Model file for the job. Use its own axes, mm. Round coordinates to 2 decimals unless told otherwise and drop trailing zeros. Loops run counter-clockwise (first coordinate to the right, second up) from the corner with the lowest first, then second, coordinate; pieces in that order, holes last. Notation, with made-up numbers: (22, 25.25) - (62, 25.25) arc R21 cw to (62, 57.25) - close; hole circle Ø10 at (-10.5, 49.25). An arc over 180 degrees is marked (long way). Use one line per item in the form item = value.
from build123d import *

# Parameters (mm, degrees)
SKETCH1_W           = 132
SKETCH1_H           = 87
BOSS_EXTRUDE1_DEPTH = 2
SKETCH2_W           = 80
SKETCH2_H           = 55
BOSS_EXTRUDE2_DEPTH = 2
SKETCH3_W           = 76
SKETCH3_H           = 51
CUT_EXTRUDE1_DEPTH  = 2
SKETCH4_W           = 70
SKETCH4_H           = 45
CUT_EXTRUDE2_DEPTH  = 2


with BuildPart() as part:
    # Sketch1 → Boss-Extrude1 (new body)
    with BuildSketch(Plane(origin=(0, 0, 0), x_dir=(1, 0, 0), z_dir=(0, 1, 0))):
        Rectangle(SKETCH1_W, SKETCH1_H)
    extrude(amount=BOSS_EXTRUDE1_DEPTH)

    # Sketch2 → Boss-Extrude2 (add)
    with BuildSketch(Plane(origin=(0, 2, 0), x_dir=(1, 0, 0), z_dir=(0, 1, 0))):
        Rectangle(SKETCH2_W, SKETCH2_H)
    extrude(amount=BOSS_EXTRUDE2_DEPTH)

    # Sketch3 → Cut-Extrude1 (cut)
    with BuildSketch(Plane(origin=(0, 4, 0), x_dir=(1, 0, 0), z_dir=(0, 1, 0))):
        Rectangle(SKETCH3_W, SKETCH3_H)
    extrude(amount=-CUT_EXTRUDE1_DEPTH, mode=Mode.SUBTRACT)

    # Sketch4 → Cut-Extrude2 (cut)
    with BuildSketch(Plane(origin=(0, 2, 0), x_dir=(1, 0, 0), z_dir=(0, 1, 0))):
        Rectangle(SKETCH4_W, SKETCH4_H)
    extrude(amount=-CUT_EXTRUDE2_DEPTH, mode=Mode.SUBTRACT)


solid = part.part
1. Wall check: probe 1 along Z at (x, y) = (27, 1.55); probe 2 along Z at (x, y) = (22.5, 3.1); probe 3 along X at (y, z) = (2.65, -4.5). Give the ranges that are in metal, low to high.
Geometry check:
probe_1 = -43.5 to -22.5, 22.5 to 43.5
probe_2 = -27.5 to -25.5, 25.5 to 27.5
probe_3 = -40 to -38, 38 to 40
2. Cut at D-D, the plane z = 24. Give the cut face in (x, y), plus the area to 3 significant figures.
Geometry check:
outline = (-66, 0) - (66, 0) - (66, 2) - (40, 2) - (40, 4) - (38, 4) - (38, 2) - (-38, 2) - (-38, 4) - (-40, 4) - (-40, 2) - (-66, 2) - close
area = 272 mm^2
3. Cut at A-A, the plane z = 1. Give the cut face in (x, y), plus the area to 3 significant figures.
Geometry check:
outline = (-66, 0) - (-35, 0) - (-35, 2) - (-38, 2) - (-38, 4) - (-40, 4) - (-40, 2) - (-66, 2) - close; (35, 0) - (66, 0) - (66, 2) - (40, 2) - (40, 4) - (38, 4) - (38, 2) - (35, 2) - close
area = 132 mm^2
4. Flat gauge pins, fed straight in: pin 1 (1.6 mm diameter, centred on y = 3, z = -6, fed in from -X); pin 2 (0.6 mm diameter, centred on y = 2.5, z = -10, fed in from +X); pin 3 (1.6 mm diameter, centred on x = -18, y = 3.5, fed in from +Z). Where does each tip first touch, or does it go through?
Geometry check:
pin_1 = -40
pin_2 = 40
pin_3 = 27.5
5. Pull direction Z, two halves, no side cores. Call faces 1 (the flat face through (-3, 4, 26)), 2 (the flat face through (-3, 2, 23)): +Z half, -Z half, draft (parallel to the pull), parting line (faces both ways), or undercut.
Geometry check:
face_1 = draft
face_2 = undercut
6. Cut at B-B, the plane y = 3.05. Give the cut face in (x, z), plus the area to 3 significant figures.
Geometry check:
outline = (-40, -27.5) - (40, -27.5) - (40, 27.5) - (-40, 27.5) - close; hole (-38, -25.5) - (38, -25.5) - (38, 25.5) - (-38, 25.5) - close
area = 524 mm^2
7. Cut at C-C, the plane x = 29.5. Give the cut face in (y, z).
Geometry check:
outline = (0, -43.5) - (2, -43.5) - (2, -27.5) - (4, -27.5) - (4, -25.5) - (2, -25.5) - (2, -22.5) - (0, -22.5) - close; (0, 22.5) - (2, 22.5) - (2, 25.5) - (4, 25.5) - (4, 27.5) - (2, 27.5) - (2, 43.5) - (0, 43.5) - close
